from build123d import *

# Parameters (mm, degrees)
F1_DEPTH = 6
F2_R     = 8.25
F2_R_2   = 8.375
F2_R_3   = 8.5
F2_R_4   = 8.625
F2_R_5   = 8.75
F2_R_6   = 8.875
F3_DEPTH = 6.001


with BuildPart() as f1:
    # F0 (on Top) → F1 (new body)
    with BuildSketch(Plane.XY):
        with BuildLine():
            Line((65, 12.5), (-65, 12.5))
            ThreePointArc((-65, 12.5), (-68.535534, 11.035534), (-70, 7.5))
            Line((-70, 7.5), (-70, -7.5))
            ThreePointArc((-70, -7.5), (-68.535534, -11.035534), (-65, -12.5))
            Line((-65, -12.5), (65, -12.5))
            ThreePointArc((65, -12.5), (68.535534, -11.035534), (70, -7.5))
            Line((70, -7.5), (70, 7.5))
            ThreePointArc((70, 7.5), (68.535534, 11.035534), (65, 12.5))
        make_face()
    extrude(amount=F1_DEPTH)

    # F2 (on face) → F3 (cut, through all)
    with BuildSketch(Plane.XY.offset(6)):
        with Locations((-56.75, 0)):
            Circle(F2_R)
        with Locations((-35.125, 0)):
            Circle(F2_R_2)
        with Locations((-13.25, 0)):
            Circle(F2_R_3)
        with Locations((8.875, 0)):
            Circle(F2_R_4)
        with Locations((31.25, 0)):
            Circle(F2_R_5)
        with Locations((53.875, 0)):
            Circle(F2_R_6)
    extrude(amount=-F3_DEPTH, mode=Mode.SUBTRACT)


solid = f1.part
Here's how the part is built. I have some questions about the finished solid (model axes, mm). Round coordinates to 2 decimals unless told otherwise and drop trailing zeros. Write each loop counter-clockwise with the first axis right and the second up, starting at its lowest first coordinate (ties: lowest second). Pieces come first, ordered by that corner, then holes.
1. Suppose I cut it at A-A (x = 31.25). List the corners of the cut face in (y, z) for me, and give its area (3 significant figures).
2. Will this pin go through, and if not, where does the flat tip stop? pin 1 Ø3 at (y, z) = (9.5, 1.5) entering from +X.
3. Suppose I cut it at D-D (x = -13.25). List the corners of the cut face in (y, z) for me.
4. If we mould it in two halves opening along X, with no side actions, what happens to faces 1 (the flat face through (-70, 0, 3)), 2 (the flat face through (-1, -12.5, 3)), 3 (the cylindrical face through (35.29, -7.76, 3.04))? For each: released by +X, released by -X, zero draft, split by the parting line, or undercut.
5. I need wall thicknesses on L1, parallel to Y at x = 56.5, z = 0.85; L2, parallel to Y at x = -56, z = 3.6; L3, parallel to X at y = -10.75, z = 1.3. Which ranges of each line are inside material? Lowest first, please.
6. Suppose I cut it at B-B (y = 0). List the corners of the cut face in (x, z) for me.
7. Suppose I cut it at C-C (z = 3.2). List the corners of the cut face in (x, y) for me (3 decimals), and give its area (3 significant figures).
Answer sheet:
1. outline: (-12.5, 0) - (-8.75, 0) - (-8.75, 6) - (-12.5, 6) - close; (8.75, 0) - (12.5, 0) - (12.5, 6) - (8.75, 6) - close
1. area: 45.0 mm2
2. pin 1: stops at x = 69.97
3. outline: (-12.5, 0) - (-8.5, 0) - (-8.5, 6) - (-12.5, 6) - close; (8.5, 0) - (12.5, 0) - (12.5, 6) - (8.5, 6) - close
4. face 1: released by -X
4. face 2: zero draft
4. face 3: undercut
5. L1: y = -12.5 to -8.48, 8.48 to 12.5
5. L2: y = -12.5 to -8.22, 8.22 to 12.5
5. L3: x = -68.8 to 68.8
6. outline: (-70, 0) - (-65, 0) - (-65, 6) - (-70, 6) - close; (-48.5, 0) - (-43.5, 0) - (-43.5, 6) - (-48.5, 6) - close; (-26.75, 0) - (-21.75, 0) - (-21.75, 6) - (-26.75, 6) - close; (-4.75, 0) - (0.25, 0) - (0.25, 6) - (-4.75, 6) - close; (17.5, 0) - (22.5, 0) - (22.5, 6) - (17.5, 6) - close; (40, 0) - (45, 0) - (45, 6) - (40, 6) - close; (62.75, 0) - (70, 0) - (70, 6) - (62.75, 6) - close
7. outline: (-70, -7.5) arc R5 ccw to (-65, -12.5) - (65, -12.5) arc R5 ccw to (70, -7.5) - (70, 7.5) arc R5 ccw to (65, 12.5) - (-65, 12.5) arc R5 ccw to (-70, 7.5) - close; hole circle Ø16.5 at (-56.75, 0); hole circle Ø16.75 at (-35.125, 0); hole circle Ø17 at (-13.25, 0); hole circle Ø17.25 at (8.875, 0); hole circle Ø17.5 at (31.25, 0); hole circle Ø17.75 at (53.875, 0)
7. area: 2,100 mm2
